Model file for the job. Use its own axes, mm. A direction names the side the tool comes from. Round coordinates to 2 decimals unless told otherwise and drop trailing zeros. Order: outer loops, then holes, each group sorted by start corner. A loop starts at its lowest first (then second) coordinate and runs counter-clockwise, first axis right, second up. Notation, with made-up numbers: (11, 59) - (42, 59) arc R20 cw to (42, 81) - close; hole circle Ø6 at (40.25, 50.5). An arc over 180 degrees is marked (long way). Use one line per item in the form item = value.
from build123d import *

# Parameters (mm, degrees)
SKETCH016_R     = 4.4
PAD004_DEPTH    = 5.71
SKETCH017_R     = 3.1
POCKET008_DEPTH = 5
SKETCH018_R     = 1.6
POCKET009_DEPTH = 7.2
CHAMFER004_SIZE = 0.5


with BuildPart() as part:
    # Sketch016 → Pad004 (new body)
    with BuildSketch(Plane.XY.offset(-7.2)):
        with Locations((-36.708672, -51.151615)):
            Circle(SKETCH016_R)
    extrude(amount=PAD004_DEPTH)

    # Sketch017 → Pocket008 (cut)
    with BuildSketch(Plane.XY.offset(-7.4)):
        with Locations((-36.718586, -51.151543)):
            Circle(SKETCH017_R)
    extrude(amount=POCKET008_DEPTH, mode=Mode.SUBTRACT)

    # Sketch018 → Pocket009 (cut)
    with BuildSketch(Plane.XY.offset(-7.2)):
        with Locations((-36.700569, -51.150215)):
            Circle(SKETCH018_R)
    extrude(amount=POCKET009_DEPTH, mode=Mode.SUBTRACT)

    # Chamfer004
    chamfer004_edges = [part.edges().sort_by_distance(p)[0] for p in [
        (-39.818586, -51.151543, -7.2),
    ]]
    chamfer(chamfer004_edges, length=CHAMFER004_SIZE)


solid = part.part
(1) Pull direction Y, two halves, no side cores. Call faces 1 (the face through (-39.816, -51.015, -4.58)), 2 (the face through (-33, -52, -7.2)), 3 (the face through (-32.51, -49.83, -4.38)): released by +Y, released by -Y, zero draft, split by the parting line, or undercut.
Report:
face_1 = undercut
face_2 = zero draft
face_3 = split by the parting line
(2) Pin check, flat tips, straight feed: pin 1 (1 mm diameter, centred on y = -53, z = -5, fed in from +X); pin 2 (1.9 mm diameter, centred on x = -37.5, y = -50, fed in from -Z); pin 3 (1.5 mm diameter, centred on y = -53.5, z = -5, fed in from -X); pin 4 (1 mm diameter, centred on y = -51.5, z = -6, fed in from -X). Stop position of each tip, or through.
Report:
pin_1 = -32.52
pin_2 = -2.4
pin_3 = -40.81
pin_4 = -41.11
(3) Tool access for faces 4 (the face through (-35, -52, -2.4)), 5 (the face through (-37, -53, -1.49)): list every direction of +Z, -Z, +X, -X, +Y, -Y with a clear straight run to the whole face (end or side of a thin tool).
Report:
face_4 = -Z
face_5 = +Z, +X, -X, +Y, -Y
(4) Slice it at B-B on z = -6.4. Give the cut face in (x, y), then the cut area to 3 significant figures.
Report:
outline = circle Ø8.8 at (-36.71, -51.15); hole circle Ø6.2 at (-36.72, -51.15)
area = 30.6 mm2
(5) Slice it at A-A on z = -2. Give the cut face in (x, y), then the cut area to 3 significant figures.
Report:
outline = circle Ø8.8 at (-36.71, -51.15); hole circle Ø3.2 at (-36.7, -51.15)
area = 52.8 mm2
(6) Probe probe 1 along Z at (x, y) = (-38.5, -52.5); probe 2 along X at (y, z) = (-51.25, -5.95); probe 3 along Y at (x, z) = (-36.5, -3.2). List the from-to ranges inside material, lowest first. Write a range as [from, to].
Report:
probe_1 = [-2.4, -1.49]
probe_2 = [-41.11, -39.82], [-33.62, -32.31]
probe_3 = [-55.55, -54.24], [-48.06, -46.76]
